Build history of the part. All positions in model axes, mm. Give positions to 0.01 mm unless a question says otherwise; leave off trailing zeros. Order: outer loops, then holes, each group sorted by start corner. A loop starts at its lowest first (then second) coordinate and runs counter-clockwise, first axis right, second up. Notation, with made-up numbers: (41, 24.25) - (64, 24.25) arc R23 cw to (64, 41.25) - close; hole circle Ø2 at (15, 72.25). An arc over 180 degrees is marked (long way). One line per item, written item: value.
```python
from build123d import *

# Parameters (mm, degrees)
RESSALTO_EXTRUS_O4_DEPTH = 5
ESBO_O2_R                = 2.5
ESBO_O2_R_2              = 3.5
ESBO_O2_R_3              = 3
CORTE_EXTRUS_O1_DEPTH    = 5


with BuildPart() as part:
    # Esboço1 → Ressalto-extrusão4 (new body)
    with BuildSketch(Plane(origin=(0, 0, 0), x_dir=(1, 0, 0), z_dir=(0, 1, 0))):
        with BuildLine():
            Line((470.007423898, -115.796995794), (602.527286899, -115.796995794))
            ThreePointArc((602.527286899, -115.796995794), (615.578185817, -112.120082753), (624.7901231, -102.17091879))
            Line((624.7901231, -102.17091879), (658.530191599, -36.129534592))
            ThreePointArc((658.530191599, -36.129534592), (660.573433908, -30.604931856), (661.267355398, -24.755611597))
            Line((661.267355398, -24.755611597), (661.267355398, 84.203004206))
            Line((661.267355398, 84.203004206), (661.267355398, 124.203004206))
            Line((661.267355398, 124.203004206), (411.267355398, 124.203004206))
            Line((411.267355398, 124.203004206), (411.267355398, 81.588187759))
            Line((411.267355398, 81.588187759), (411.267355398, -27.370428044))
            ThreePointArc((411.267355398, -27.370428044), (412.010540804, -33.420795447), (414.195911055, -39.11143927))
            Line((414.195911055, -39.11143927), (447.935979555, -102.53800702))
            ThreePointArc((447.935979555, -102.53800702), (457.133521627, -112.227409704), (470.007423898, -115.796995794))
        make_face()
    extrude(amount=RESSALTO_EXTRUS_O4_DEPTH)

    # Esboço2 → Corte-extrusão1 (cut)
    with BuildSketch(Plane(origin=(0, 5, 0), x_dir=(1, 0, 0), z_dir=(0, 1, 0))):
        with Locations(Location((571.267355398, -100.796995794, 0), (0, 0, 270))):
            Circle(ESBO_O2_R)
        with Locations(Location((501.267355398, -100.796995794, 0), (0, 0, 270))):
            Circle(ESBO_O2_R)
        with Locations(Location((646.267355398, 69.203004206, 0), (0, 0, 270))):
            Circle(ESBO_O2_R)
        with Locations(Location((426.267355398, 69.203004206, 0), (0, 0, 270))):
            Circle(ESBO_O2_R)
        with Locations(Location((536.267355398, -99.396995794, 0), (0, 0, 270))):
            Circle(ESBO_O2_R_2)
        with Locations(Location((536.267355398, -89.796995794, 0), (0, 0, 270))):
            Circle(ESBO_O2_R_3)
        with Locations(Location((644.867355398, 104.203004206, 0), (0, 0, 270))):
            Circle(ESBO_O2_R_2)
        with Locations(Location((635.267355398, 104.203004206, 0), (0, 0, 270))):
            Circle(ESBO_O2_R_3)
        with Locations(Location((427.667355398, 104.203004206, 0), (0, 0, 270))):
            Circle(ESBO_O2_R_2)
        with Locations(Location((437.267355398, 104.203004206, 0), (0, 0, 270))):
            Circle(ESBO_O2_R_3)
    extrude(amount=-CORTE_EXTRUS_O1_DEPTH, mode=Mode.SUBTRACT)


solid = part.part
```
(1) Slice it at A-A, the plane y = 3.15. Count the separate pieces of the cut face and the enclosed holes in it, and give its area (3 significant figures).
Completed:
separate pieces: 1
enclosed holes: 10
area: 56,000 mm²
(2) Pin check, flat tips, straight feed: P1, Ø6.5, axis at x = 644.87, z = -104.2, coming from the -Y side; P2, Ø1.5, axis at y = 2.5, z = 65.5, coming from the +X side. Stop position of each tip, or through.
Completed:
P1: through
P2: x = 643.91
(3) Pull direction X, two halves, no side cores. Call faces 1 (the face through (535, 5, -6)), 2 (the face through (440.242, 2.535, -104.594)), 3 (the face through (456.97, 2.46, 112.13)): +X half, -X half, draft (parallel to the pull), parting line (faces both ways), or undercut.
Completed:
face 1: draft
face 2: undercut
face 3: -X half
(4) Drill centre lines: line 1 (X direction, y = 3.25, z = 99); line 2 (Z direction, x = 501, y = 2.65); line 3 (X direction, y = 4.4, z = 98.5). Where is each one in solid material? Low to high.
Completed:
line 1: 446.05 to 499.53, 503.01 to 532.79, 539.74 to 569.53, 573.01 to 626.41
line 2: -124.2 to 98.31, 103.28 to 115.8
line 3: 445.79 to 500.28, 502.25 to 532.88, 539.65 to 570.28, 572.25 to 626.67
(5) Slice it at B-B, the plane z = 82. Give the cut face in (x, y).
Completed:
outline: (437.01, 0) - (635.1, 0) - (635.1, 5) - (437.01, 5) - close
